Here's how the part is built. I have some questions about the finished solid (model axes, mm). Round coordinates to 2 decimals unless told otherwise and drop trailing zeros. Loops run counter-clockwise (first coordinate to the right, second up) from the corner with the lowest first, then second, coordinate; pieces in that order, holes last. Notation, with made-up numbers: M -1,-38.5 L 34,-38.5 A30 cw 34,-13.5 Z; hole C 32,25 d2. An arc over 180 degrees is marked long. Answer as a JSON object with one key per item and string values.
from build123d import *

# Parameters (mm, degrees)
SKETCH1_W           = 10
SKETCH1_H           = 19
SKETCH1_R           = 2.525
BOSS_EXTRUDE1_DEPTH = 24.9
SKETCH2_R           = 2.65
CUT_EXTRUDE1_DEPTH  = 2.5
FILLET1_R           = 0.2
CHAMFER1_SIZE       = 0.2


with BuildPart() as part:
    # Sketch1 → Boss-Extrude1 (new body, symmetric)
    with BuildSketch(Plane(origin=(0, 0, 0), x_dir=(1, 0, 0), z_dir=(0, 1, 0))):
        Rectangle(SKETCH1_W, SKETCH1_H)
        with Locations((-0.5, 0)):
            Circle(SKETCH1_R, mode=Mode.SUBTRACT)
    extrude(amount=BOSS_EXTRUDE1_DEPTH, both=True)

    # Sketch2 → Cut-Extrude1 (cut)
    with BuildSketch(Plane(origin=(5, 0, 0), x_dir=(0, 0, -1), z_dir=(1, 0, 0))):
        with Locations((3.5, 0)):
            Circle(SKETCH2_R)
    extrude(amount=-CUT_EXTRUDE1_DEPTH, mode=Mode.SUBTRACT)

    # Fillet1
    fillet1_edges = [part.edges().sort_by_distance(p)[0] for p in [
        (5, 24.9, 0),
        (0, 24.9, -9.5),
        (-5, 24.9, 0),
        (0, -24.9, -9.5),
        (5, -24.9, 0),
        (0, -24.9, 9.5),
        (-5, -24.9, 0),
        (-5, 0, -9.5),
        (5, 0, -9.5),
        (5, 0, 9.5),
        (-5, 0, 9.5),
        (0, 24.9, 9.5),
    ]]
    fillet(fillet1_edges, radius=FILLET1_R)

    # Chamfer1
    chamfer1_edges = [part.edges().sort_by_distance(p)[0] for p in [
        (-3.025, 24.9, 0),
        (5, 0, -0.85),
    ]]
    chamfer(chamfer1_edges, length=CHAMFER1_SIZE)


solid = part.part
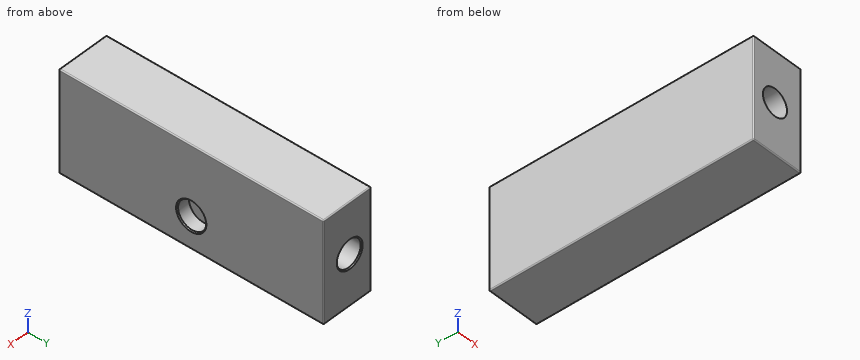
Item 1: I want a section at A-A on y = 0. List the corners of the cut face in (x, z) for me (3 decimals), plus the area to 3 significant figures.
Solution:
{"outline": "M -5,-9.3 A0.2 ccw -4.8,-9.5 L 4.8,-9.5 A0.2 ccw 5,-9.3 L 5,-6.35 L 4.8,-6.15 L 2.5,-6.15 L 2.5,-0.85 L 4.8,-0.85 L 5,-0.65 L 5,9.3 A0.2 ccw 4.8,9.5 L -4.8,9.5 A0.2 ccw -5,9.3 Z; hole C -0.5,0 d5.05", "area": "157 mm2"}
Item 2: I want a section at C-C on x = -0.5. List the corners of the cut face in (y, z) for me (3 decimals), plus the area to 3 significant figures.
Solution:
{"outline": "M -24.9,-9.3 A0.2 ccw -24.7,-9.5 L 24.7,-9.5 A0.2 ccw 24.9,-9.3 L 24.9,-2.725 L 24.7,-2.525 L -24.9,-2.525 Z; M -24.9,2.525 L 24.7,2.525 L 24.9,2.725 L 24.9,9.3 A0.2 ccw 24.7,9.5 L -24.7,9.5 A0.2 ccw -24.9,9.3 Z", "area": "695 mm2"}
Item 3: If I drill on L1, parallel to Y at x = 3.4, z = -3.5; L2, parallel to X at y = -13, z = 0 (3 decimals); L3, parallel to Z at x = -0.5, y = -2.5 (3 decimals), over which ranges is the centre line in solid material (lowest first)? Write a range as from..to.
Solution:
{"L1": "y = -24.9..-2.65, 2.65..24.9", "L2": "x = -5..-3.025, 2.025..5", "L3": "z = -9.5..-2.525, 2.525..9.5"}
Item 4: I want a section at B-B on z = 0. List the corners of the cut face in (x, y) for me (3 decimals).
Solution:
{"outline": "M -5,-24.7 A0.2 ccw -4.8,-24.9 L -3.025,-24.9 L -3.025,24.7 L -3.225,24.9 L -4.8,24.9 A0.2 ccw -5,24.7 Z; M 2.025,-24.9 L 4.8,-24.9 A0.2 ccw 5,-24.7 L 5,24.7 A0.2 ccw 4.8,24.9 L 2.225,24.9 L 2.025,24.7 Z"}
Item 5: I want a section at D-D on z = -3.5. List the corners of the cut face in (x, y) for me, plus the area to 3 significant figures.
Solution:
{"outline": "M -5,-24.7 A0.2 ccw -4.8,-24.9 L 4.8,-24.9 A0.2 ccw 5,-24.7 L 5,-2.85 L 4.8,-2.65 L 2.5,-2.65 L 2.5,2.65 L 4.8,2.65 L 5,2.85 L 5,24.7 A0.2 ccw 4.8,24.9 L -4.8,24.9 A0.2 ccw -5,24.7 Z", "area": "485 mm2"}
Item 6: For P1, Ø4, axis at x = -0.5, z = 0, coming from the -Y side; P2, Ø5, axis at y = 0, z = -3.5, coming from the +X side, each with a flat end and sliding along its axis, tell me the tip position at first contact or that it passes through.
Solution:
{"P1": "passes through", "P2": "stops at x = 2.5"}
